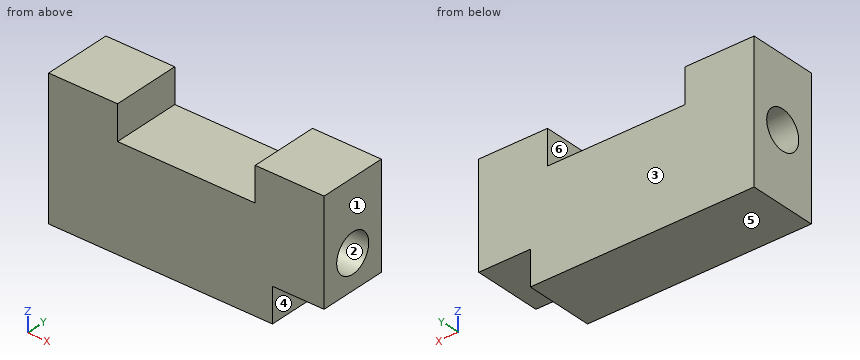
from build123d import *

# Parameters (mm, degrees)
F0_W     = 101.6
F0_H     = 50.8
F1_DEPTH = 25.4
F2_W     = 50.8
F2_H     = 12.7
F3_DEPTH = 25.401
F4_W     = 25.4
F4_H     = 12.7
F5_DEPTH = 19.05
F6_R     = 7.110031
F7_DEPTH = 101.601


with BuildPart() as f1:
    # F0 (on Front) → F1 (new body)
    with BuildSketch(Plane.XZ):
        Rectangle(F0_W, F0_H)
    extrude(amount=F1_DEPTH)

    # F2 (on face) → F3 (cut, through all)
    with BuildSketch(Plane.XZ.offset(25.4)):
        with Locations((0, 19.05)):
            Rectangle(F2_W, F2_H)
    extrude(amount=-F3_DEPTH, mode=Mode.SUBTRACT)

    # F4 (on face) → F5 (cut)
    with BuildSketch(Plane.YZ.offset(50.8)):
        with Locations((-12.7, -19.05)):
            Rectangle(F4_W, F4_H)
    extrude(amount=-F5_DEPTH, mode=Mode.SUBTRACT)

    # F6 (on face) → F7 (cut, through all)
    with BuildSketch(Plane.YZ.offset(50.8)):
        with Locations((-12.7, 0)):
            Circle(F6_R)
    extrude(amount=-F7_DEPTH, mode=Mode.SUBTRACT)


solid = f1.part
Verification items for the finished model (mm, model axes). Face numbers are marked on the shaded views. A direction names the side the tool comes from. Coordinates: 2 decimals unless noted, no trailing zeros. Order: outer loops, then holes, each group sorted by start corner. A loop starts at its lowest first (then second) coordinate and runs counter-clockwise, first axis right, second up. Notation, with made-up numbers: M 11,38.25 L 38,38.25 A10 cw 38,52.25 Z; hole C 1,40.5 d3. An arc over 180 degrees is marked long. Return JSON: item names as keys, results as strings.
1) Thickness scan on L1, parallel to Z at x = -16.5, y = -12.7; L2, parallel to X at y = -19.75, z = -19; L3, parallel to Z at x = 34, y = -7.5. Record the ranges inside material, lowest first. Write a range as [from, to].
Answer list:
{"L1": "[-25.4, -7.11], [7.11, 12.7]", "L2": "[-50.8, 31.75]", "L3": "[-12.7, -4.85], [4.85, 25.4]"}
2) Gauge pin test, flat ends, axial feed: pin 1 (6 mm diameter, centred on x = 16, z = 15.5, fed in from +Y); pin 2 (6 mm diameter, centred on x = 18.5, y = -19, fed in from +Z); pin 3 (10 mm diameter, centred on y = -19, z = -22, fed in from +X); pin 4 (9.5 mm diameter, centred on x = 41.5, y = -12.5, fed in from -Z). Record the tip position at first contact, or that the pin passes through.
Answer list:
{"pin 1": "y = 0", "pin 2": "z = 12.7", "pin 3": "x = 31.75", "pin 4": "z = -12.7"}
3) Access from +Z, -Z, +X, -X, +Y, -Y to the whole of each face (thin tool, end or side, straight path). Record for the marked faces 4, 5 and 6.
Answer list:
{"face 4": "-Z, +X, +Y, -Y", "face 5": "-Z, +X, -X, +Y, -Y", "face 6": "+Z, +Y, -Y"}
4) Cross-section at B-B, the plane z = 0. Record the boundary of the cut face in (x, y).
Answer list:
{"outline": "M -50.8,-25.4 L 50.8,-25.4 L 50.8,-19.81 L -50.8,-19.81 Z; M -50.8,-5.59 L 50.8,-5.59 L 50.8,0 L -50.8,0 Z"}
5) Cross-section at A-A, the plane y = -12.7. Record the boundary of the cut face in (x, z).
Answer list:
{"outline": "M -50.8,-25.4 L 31.75,-25.4 L 31.75,-12.7 L 50.8,-12.7 L 50.8,-7.11 L -50.8,-7.11 Z; M -50.8,7.11 L 50.8,7.11 L 50.8,25.4 L 25.4,25.4 L 25.4,12.7 L -25.4,12.7 L -25.4,25.4 L -50.8,25.4 Z"}
6) Cross-section at C-C, the plane x = 30. Record the boundary of the cut face in (y, z), and give its area (3 significant figures).
Answer list:
{"outline": "M -25.4,-25.4 L 0,-25.4 L 0,25.4 L -25.4,25.4 Z; hole C -12.7,0 d14.22", "area": "1,130 mm2"}
7) Cross-section at D-D, the plane y = -21. Record the boundary of the cut face in (x, z), and give its area (3 significant figures).
Answer list:
{"outline": "M -50.8,-25.4 L 31.75,-25.4 L 31.75,-12.7 L 50.8,-12.7 L 50.8,25.4 L 25.4,25.4 L 25.4,12.7 L -25.4,12.7 L -25.4,25.4 L -50.8,25.4 Z", "area": "4,270 mm2"}
8) Release check for a two-part mould opening along Y. For the marked faces 1, 2 and 3 record: +Y half, -Y half, draft (parallel to the pull), parting line (faces both ways), or undercut.
Answer list:
{"face 1": "draft", "face 2": "undercut", "face 3": "+Y half"}
